Study the drawing (mm; zero at the part's minimum x, y, z) and answer. A direction names the side the tool comes from. Round coordinates to 2 decimals unless told otherwise and drop trailing zeros. Order: outer loops, then holes, each group sorted by start corner. A loop starts at its lowest first (then second) coordinate and runs counter-clockwise, first axis right, second up. Notation, with made-up numbers: M 28,86 L 36,86 A26 ccw 36,122 Z; hole C 35.25,87 d8. An arc over 180 degrees is marked long. Put each result on its own line as item: value. Start each with the question number.
1. Which of the six approach directions +Z, -Z, +X, -X, +Y, -Y give full straight-line access (tool end or side, diameter ignored) to the marked faces 1, 2 and 3?
2. The mould has two halves that part along X. Classify the marked faces 4, 5 and 6: +X half, -X half, draft (parallel to the pull), parting line (faces both ways), or undercut.
3. The part is cut by section B-B (z = 3). Give the vertices of the cut face in (x, y), then the cut area to 3 significant figures.
4. The part is cut by section A-A (y = 7). Give the vertices of the cut face in (x, z).
5. The part is cut by section C-C (x = 10.6). Give the vertices of the cut face in (y, z).
6. Each of these flat-tipped pins is pushed along its axis until it touches: pin 1 Ø3 at (x, y) = (12, 25.5) entering from -Z; pin 2 Ø1 at (x, y) = (7, 25) entering from -Z (1 decimal); pin 3 Ø2 at (y, z) = (14.5, 6) entering from -X. Where does it stop, or does it pass through?
7. Consider line 1 (X direction, y = 13, z = 5.5); line 2 (Y direction, x = 10.6, z = 4); line 3 (Z direction, x = 14.25, y = 14). Determine where each line is inside the solid, lowest interval first.
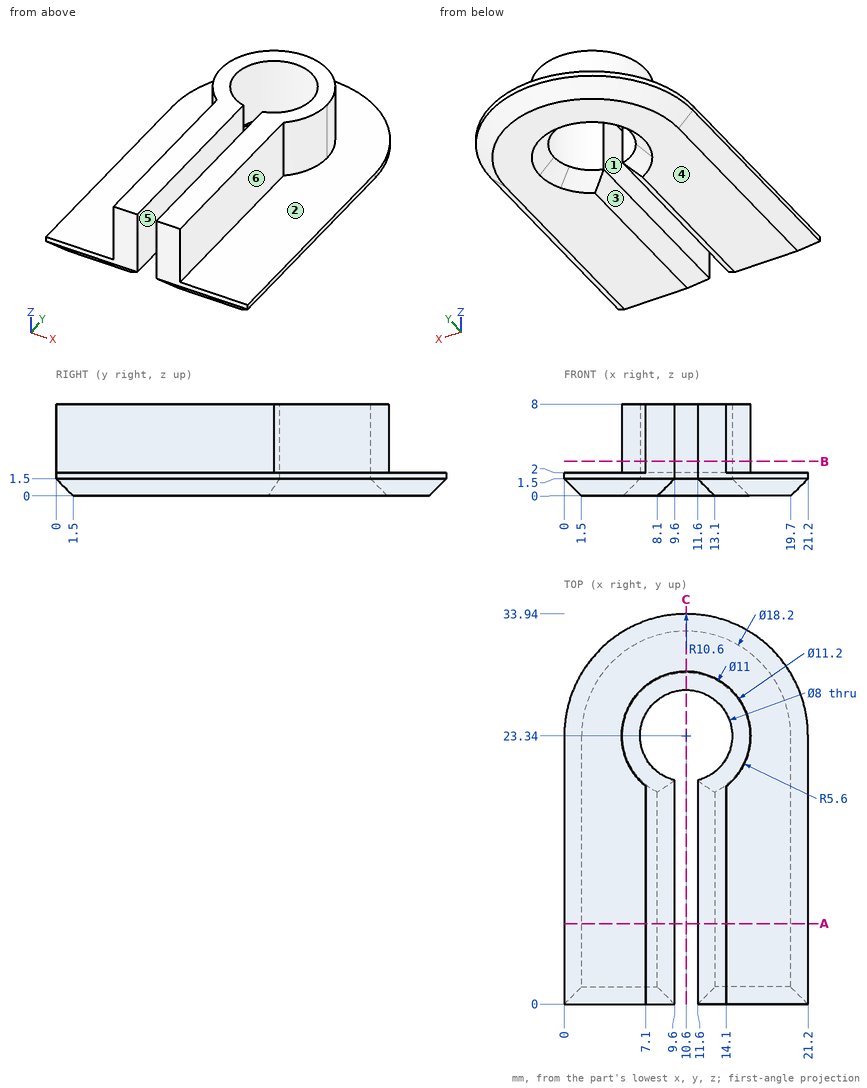
Resolved:
1. face 1: +Z, -Z, -Y
1. face 2: +Z
1. face 3: -Z, -Y
2. face 4: draft
2. face 5: undercut
2. face 6: +X half
3. outline: M 7.1,0 L 9.6,0 L 9.6,19.47 A4 cw long 11.6,19.47 L 11.6,0 L 14.1,0 L 14.1,18.97 A5.6 ccw long 7.1,18.97 Z
3. area: 136 mm2
4. outline: M 0,1.5 L 1.5,0 L 8.1,0 L 9.6,1.5 L 9.6,8 L 7.1,8 L 7.1,2 L 0,2 Z; M 11.6,1.5 L 13.1,0 L 19.7,0 L 21.2,1.5 L 21.2,2 L 14.1,2 L 14.1,8 L 11.6,8 Z
5. outline: M 27.34,1.5 L 28.84,0 L 32.44,0 L 33.94,1.5 L 33.94,2 L 28.94,2 L 28.94,8 L 27.34,8 Z
6. pin 1: z = 1.43
6. pin 2: z = 1
6. pin 3: x = 7.1
7. line 1: 7.1 to 9.6, 11.6 to 14.1
7. line 2: 27.34 to 28.94
7. line 3: 0 to 2
